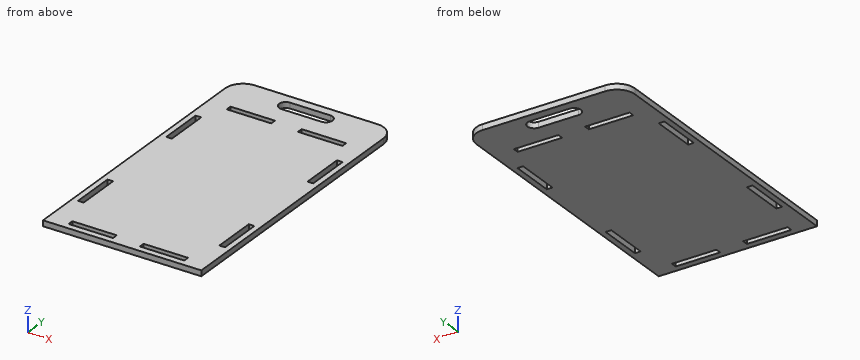
from build123d import *

# Parameters (mm, degrees)
F0_W     = 12.7
F0_H     = 100
F0_W_2   = 100
F0_H_2   = 12.7
F1_DEPTH = 12.7
F3_DEPTH = 12.7


with BuildPart() as f1:
    # F0 (on Top) → F1 (new body)
    with BuildSketch(Plane.XY):
        with BuildLine():
            Line((-177.9, -330), (177.9, -330))
            Line((177.9, -330), (177.9, 290))
            ThreePointArc((177.9, 290), (166.184271, 318.284271), (137.9, 330))
            Line((137.9, 330), (-137.9, 330))
            ThreePointArc((-137.9, 330), (-166.184271, 318.284271), (-177.9, 290))
            Line((-177.9, 290), (-177.9, -330))
        make_face()
        with Locations((-158.85, -180)):
            Rectangle(F0_W, F0_H, mode=Mode.SUBTRACT)
        with Locations((-80, -309.05)):
            Rectangle(F0_W_2, F0_H_2, mode=Mode.SUBTRACT)
        with Locations((80, -309.05)):
            Rectangle(F0_W_2, F0_H_2, mode=Mode.SUBTRACT)
        with Locations((158.85, -180)):
            Rectangle(F0_W, F0_H, mode=Mode.SUBTRACT)
        with Locations((-158.85, 120)):
            Rectangle(F0_W, F0_H, mode=Mode.SUBTRACT)
        with Locations((-80, 229.05)):
            Rectangle(F0_W_2, F0_H_2, mode=Mode.SUBTRACT)
        with Locations((158.85, 120)):
            Rectangle(F0_W, F0_H, mode=Mode.SUBTRACT)
        with Locations((80, 229.05)):
            Rectangle(F0_W_2, F0_H_2, mode=Mode.SUBTRACT)
    extrude(amount=F1_DEPTH)

    # F2 (on face) → F3 (cut, through all)
    with BuildSketch(Plane.XY.offset(12.7)):
        with BuildLine():
            ThreePointArc((-60, 295), (-55.606602, 284.393398), (-45, 280))
            Line((-45, 280), (45, 280))
            ThreePointArc((45, 280), (55.606602, 284.393398), (60, 295))
            ThreePointArc((60, 295), (55.606602, 305.606602), (45, 310))
            Line((45, 310), (-45, 310))
            ThreePointArc((-45, 310), (-55.606602, 305.606602), (-60, 295))
        make_face()
    extrude(amount=-F3_DEPTH, mode=Mode.SUBTRACT)


solid = f1.part
Design review of the part built by this model. Coordinates are the model's own, in mm. Round coordinates to 2 decimals unless told otherwise and drop trailing zeros. Loops run counter-clockwise (first coordinate to the right, second up) from the corner with the lowest first, then second, coordinate; pieces in that order, holes last. Notation, with made-up numbers: M -17.5,86.25 L 1.5,86.25 A34 ccw 1.5,125.25 Z; hole C 19.5,88.5 d2. An arc over 180 degrees is marked long. Answer as a JSON object with one key per item and string values.
Item 1: Clearance check with flat-ended pins moving along their axes: P1, Ø4, axis at x = 158.5, z = 8.5, coming from the +Y side; P2, Ø5, axis at x = 140.5, z = 6, coming from the +Y side. State where each tip first meets the part, or that it passes through.
Answer sheet:
{"P1": "stops at y = 325.41", "P2": "stops at y = 330"}
Item 2: Wall thickness on L1, parallel to Y at x = -88, z = 2.5; L2, parallel to Y at x = 46, z = 7; L3, parallel to X at y = -219, z = 10.25: over which ranges is each line inside the solid? List them lowest first. Write a range as from..to.
Answer sheet:
{"L1": "y = -330..-315.4, -302.7..222.7, 235.4..330", "L2": "y = -330..-315.4, -302.7..222.7, 235.4..280.03, 309.97..330", "L3": "x = -177.9..-165.2, -152.5..152.5, 165.2..177.9"}
Item 3: We need section B-B on y = -217.5. Give the boundary of the cut face in (x, z).
Answer sheet:
{"outline": "M -177.9,0 L -165.2,0 L -165.2,12.7 L -177.9,12.7 Z; M -152.5,0 L 152.5,0 L 152.5,12.7 L -152.5,12.7 Z; M 165.2,0 L 177.9,0 L 177.9,12.7 L 165.2,12.7 Z"}
Item 4: We need section A-A on x = -68.5. Give the boundary of the cut face in (y, z), and give its area (3 significant figures).
Answer sheet:
{"outline": "M -330,0 L -315.4,0 L -315.4,12.7 L -330,12.7 Z; M -302.7,0 L 222.7,0 L 222.7,12.7 L -302.7,12.7 Z; M 235.4,0 L 330,0 L 330,12.7 L 235.4,12.7 Z", "area": "8,060 mm^2"}
Item 5: We need section C-C on z = 8. State how many separate pieces and enclosed holes the cut face has, and give its area (3 significant figures).
Answer sheet:
{"separate pieces": "1", "enclosed holes": "9", "area": "221,000 mm^2"}
